from build123d import *

# Parameters (mm, degrees)
SKETCH1_R           = 43.5
SKETCH1_R_2         = 1.65
SKETCH1_R_3         = 12.5
BOSS_EXTRUDE1_DEPTH = 3


with BuildPart() as part:
    # Sketch1 → Boss-Extrude1 (new body)
    with BuildSketch(Plane.XY):
        Circle(SKETCH1_R)
        with Locations((-12.5, -2.5)):
            Circle(SKETCH1_R_2, mode=Mode.SUBTRACT)
        with Locations((12.5, -2.5)):
            Circle(SKETCH1_R_2, mode=Mode.SUBTRACT)
        with Locations((12.5, 22.5)):
            Circle(SKETCH1_R_2, mode=Mode.SUBTRACT)
        with Locations((-12.5, 22.5)):
            Circle(SKETCH1_R_2, mode=Mode.SUBTRACT)
        with Locations((0, 10)):
            Circle(SKETCH1_R_3, mode=Mode.SUBTRACT)
    extrude(amount=BOSS_EXTRUDE1_DEPTH)


solid = part.part
Geometry: final body of the model. Coordinates: model frame, mm. Give positions to 0.01 mm unless a question says otherwise; leave off trailing zeros. Loops run counter-clockwise (first coordinate to the right, second up) from the corner with the lowest first, then second, coordinate; pieces in that order, holes last. Notation, with made-up numbers: M -35,39 L 8,39 A20 ccw 8,59 Z; hole C 3.25,51 d11. An arc over 180 degrees is marked long. Put each result on its own line as item: value. Start each with the question number.
1) Cut plane D-D (y = 30). Output: boundary loops of the cut face in (x, z).
2) Pull-direction query (X, two-part tool) for faces 1 (the cylindrical face through (-5.66, 43.13, 1.48)), 2 (the flat face through (-1, -9, 0)), 3 (the cylindrical face through (14.024, -3.132, 1.479)); classes: pulls with the +X half, pulls with the -X half, needs draft (parallel to the pull), parting line crosses it, or undercut.
3) Cut plane C-C (z = 2.15). Output: boundary loops of the cut face in (x, y).
4) Ray query, line 1 along X through (y, z) = (-3.5, 1.5); line 2 along X through (y, z) = (5.5, 1.6); line 3 along Y through (x, z) = (-25.5, 0.35). Return the intervals inside material, ascending.
5) Cut plane B-B (y = 10). Output: boundary loops of the cut face in (x, z).
6) Contact query for a flat-ended pin moving along its axis: pin 1 (1 mm diameter, centred on x = -25, z = 2, fed in from -Y). Output: stop coordinate, or through.
7) Cut plane A-A (x = 0). Output: boundary loops of the cut face in (y, z).
Verdict:
1. outline: M -31.5,0 L 31.5,0 L 31.5,3 L -31.5,3 Z
2. face 1: parting line crosses it
2. face 2: needs draft
2. face 3: undercut
3. outline: C 0,0 d87; hole C -12.5,-2.5 d3.3; hole C -12.5,22.5 d3.3; hole C 0,10 d25; hole C 12.5,-2.5 d3.3; hole C 12.5,22.5 d3.3
4. line 1: -43.36 to -13.81, -11.19 to 11.19, 13.81 to 43.36
4. line 2: -43.15 to -11.66, 11.66 to 43.15
4. line 3: -35.24 to 35.24
5. outline: M -42.33,0 L -12.5,0 L -12.5,3 L -42.33,3 Z; M 12.5,0 L 42.33,0 L 42.33,3 L 12.5,3 Z
6. pin 1: y = -35.94
7. outline: M -43.5,0 L -2.5,0 L -2.5,3 L -43.5,3 Z; M 22.5,0 L 43.5,0 L 43.5,3 L 22.5,3 Z
